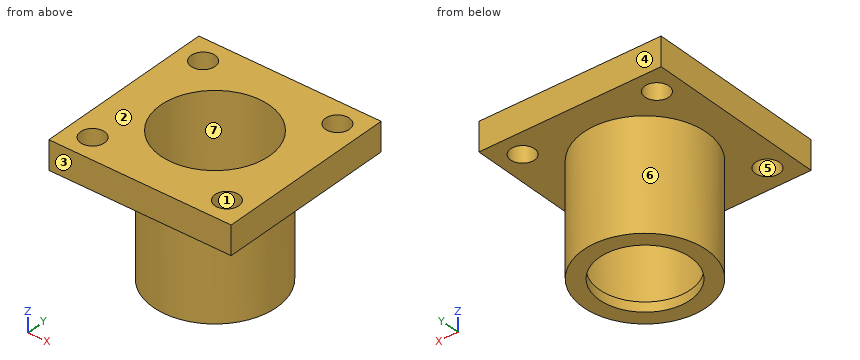
from build123d import *

# Parameters (mm, degrees)
SKETCH001_R   = 9.5
POCKET_DEPTH  = 2
SKETCH002_W   = 38
SKETCH002_H   = 38
SKETCH002_R   = 11.35
SKETCH002_R_2 = 2.5
PAD_DEPTH     = 6


with BuildPart() as part:
    # Sketch → Revolution (revolve)
    with BuildSketch(Plane.XZ):
        Polygon((-11.35, 27), (-11.35, 2), (0, 2), (0, 0), (-12.85, 0), (-12.85, 27), (-12.85, 29), (-11.35, 29), align=None)
    revolve(axis=Axis((0, 0, 0), (0, 0, 1)))

    # Sketch001 (on Face3 of Revolution) → Pocket (cut)
    with BuildSketch(Plane(origin=(0, 0, 0), x_dir=(1, 0, 0), z_dir=(0, 0, -1))):
        Circle(SKETCH001_R)
    extrude(amount=-POCKET_DEPTH, mode=Mode.SUBTRACT)

    # Sketch002 (on Face4 of Pocket) → Pad (join)
    with BuildSketch(Plane(origin=(0, 0, 29), x_dir=(-1, 0, 0), z_dir=(0, 0, 1))):
        Rectangle(SKETCH002_W, SKETCH002_H)
        Circle(SKETCH002_R, mode=Mode.SUBTRACT)
        with Locations((-14, 14)):
            Circle(SKETCH002_R_2, mode=Mode.SUBTRACT)
        with Locations((14, 14)):
            Circle(SKETCH002_R_2, mode=Mode.SUBTRACT)
        with Locations((14, -14)):
            Circle(SKETCH002_R_2, mode=Mode.SUBTRACT)
        with Locations((-14, -14)):
            Circle(SKETCH002_R_2, mode=Mode.SUBTRACT)
    extrude(amount=-PAD_DEPTH)


solid = part.part
Work out the finished part from the listing and answer in its coordinate system (mm). Face numbers are marked on the shaded views. A direction names the side the tool comes from. Give positions to 0.01 mm unless a question says otherwise; leave off trailing zeros. Loops run counter-clockwise (first coordinate to the right, second up) from the corner with the lowest first, then second, coordinate; pieces in that order, holes last. Notation, with made-up numbers: (22, 25) -> (60, 25) arc R7 ccw to (60, 37) -> close; hole circle Ø11 at (-33.75, 55.25). An arc over 180 degrees is marked (long way). Use a Markdown table: item, result. Add a question column.
1) The part is cut by section B-B, the plane x = 14. Determine the outline of the cut face in (y, z), plus the area to 3 significant figures.
2) For a pull along Y with two mould halves and no side action, classify the marked faces 1, 2, 3 and 4 as +Y half, -Y half, draft (parallel to the pull), parting line (faces both ways), or undercut.
3) Each of these flat-tipped pins is pushed along its axis until it touches: P1, Ø6.5, axis at x = 14, y = 14, coming from the -Z side; P2, Ø10, axis at y = -12, z = 17.5, coming from the -X side; P3, Ø4, axis at x = 0.5, z = 4, coming from the -Y side. Where does it stop, or does it pass through?
4) Consider line 1 along Y through (x, z) = (14, 24.3); line 2 along X through (y, z) = (-15.5, 24). Determine where each line is inside the solid, lowest interval first.
5) The part is cut by section A-A, the plane y = 0. Determine the outline of the cut face in (x, z), plus the area to 3 significant figures.
6) Which of the six approach directions +Z, -Z, +X, -X, +Y, -Y give full straight-line access (tool end or side, diameter ignored) to the marked faces 5, 6 and 7?
Reported:
| question | item | result |
|---|---|---|
| 1 | outline | (-19, 23) -> (-16.5, 23) -> (-16.5, 29) -> (-19, 29) -> close; (-11.5, 23) -> (11.5, 23) -> (11.5, 29) -> (-11.5, 29) -> close; (16.5, 23) -> (19, 23) -> (19, 29) -> (16.5, 29) -> close |
| 1 | area | 168 mm^2 |
| 2 | face 1 | undercut |
| 2 | face 2 | draft |
| 2 | face 3 | -Y half |
| 2 | face 4 | +Y half |
| 3 | P1 | stops at z = 23 |
| 3 | P2 | stops at x = -10.78 |
| 3 | P3 | stops at y = -12.85 |
| 4 | line 1 | y = -19 to -16.5, -11.5 to 11.5, 16.5 to 19 |
| 4 | line 2 | x = -19 to -16, -12 to 12, 16 to 19 |
| 5 | outline | (-19, 23) -> (-12.85, 23) -> (-12.85, 0) -> (-9.5, 0) -> (-9.5, 2) -> (-11.35, 2) -> (-11.35, 29) -> (-19, 29) -> close; (9.5, 0) -> (12.85, 0) -> (12.85, 23) -> (19, 23) -> (19, 29) -> (11.35, 29) -> (11.35, 2) -> (9.5, 2) -> close |
| 5 | area | 168 mm^2 |
| 6 | face 5 | +Z, -Z |
| 6 | face 6 | -Z |
| 6 | face 7 | +Z |
